For this review, take the finished solid that the model builds, in its own axes (mm). Face numbers are marked on the shaded views. Coordinates: 2 decimals unless noted, no trailing zeros. Write each loop counter-clockwise with the first axis right and the second up, starting at its lowest first coordinate (ties: lowest second). Pieces come first, ordered by that corner, then holes. Notation, with made-up numbers: (73.5, 17.25) -> (116.5, 17.25) arc R23 ccw to (116.5, 33.25) -> close; hole circle Ø4 at (32, 14.5). An arc over 180 degrees is marked (long way). Put each result on its own line as item: value. Start each with the question number.
Item 1: Consider section A-A on x = 92. Give the boundary of the cut face in (y, z) (1 decimal).
Item 2: Consider section D-D on z = 3.5. Give the boundary of the cut face in (x, y).
Item 3: To check wall thickness, follow L1, parallel to X at y = 45.5, z = -2 (3 decimals); L2, parallel to X at y = 52.5, z = -0.75; L3, parallel to Y at x = 103, z = -2.25. State the ranges of each line that lie inside material, in increasing order.
Item 4: Consider section C-C on y = 53. Give the boundary of the cut face in (x, z) (1 decimal), and give its area (3 significant figures).
Item 5: Consider section B-B on y = 42.5. Give the boundary of the cut face in (x, z) (1 decimal).
Item 6: The part is to be moulded in two halves that separate along Z. For the marked faces 1 and 2, say which applies: +Z half, -Z half, draft (parallel to the pull), parting line (faces both ways), or undercut.
Item 7: Insertion check: P1, Ø1, axis at x = 99, z = 0.5, coming from the -Y side; P2, Ø13, axis at x = 95.86, y = 45.47, coming from the -Z side; P3, Ø4, axis at y = 31, z = 2, coming from the +X side. Each pin has a flat end and moves straight along its axis. Give the tip position at first contact, or say it passes through.
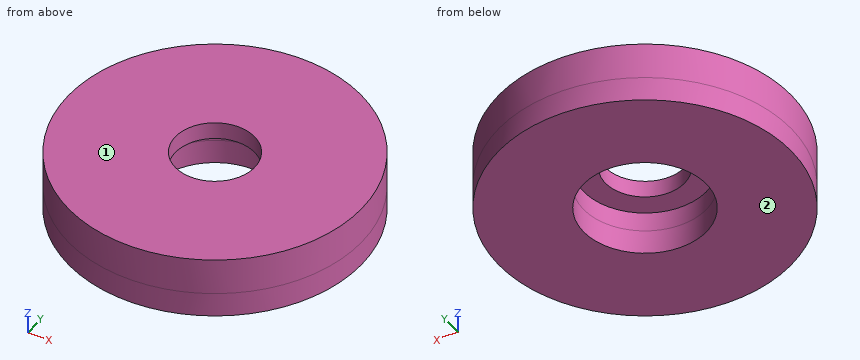
```python
from build123d import *

# Parameters (mm, degrees)
SKETCH1_R               = 19.05
SKETCH1_R_2             = 8.001
BOSS_EXTRUDE1_DEPTH     = 3.175
SKETCH2_R               = 19.05
BOSS_EXTRUDE2_DEPTH     = 4.7625
F_3_8_CLEARANCE_HOLE1_D = 10.31748
SKETCH6_R               = 8.001
CUT_EXTRUDE1_DEPTH      = 2.54


with BuildPart() as part:
    # Sketch1 → Boss-Extrude1 (new body)
    with BuildSketch(Plane.XY):
        with Locations((95.864074702, 45.465579041)):
            Circle(SKETCH1_R)
        with Locations((95.864074702, 45.465579041)):
            Circle(SKETCH1_R_2, mode=Mode.SUBTRACT)
    extrude(amount=-BOSS_EXTRUDE1_DEPTH)

    # Sketch2 → Boss-Extrude2 (add)
    with BuildSketch(Plane.XY):
        with Locations((95.864074702, 45.465579041)):
            Circle(SKETCH2_R)
    extrude(amount=BOSS_EXTRUDE2_DEPTH)

    # 3/8 Clearance Hole1 (through all)
    with Locations(Plane.XY.offset(4.7625)):
        with Locations((95.864074702, 45.465579041)):
            Hole(F_3_8_CLEARANCE_HOLE1_D / 2)

    # Sketch6 → Cut-Extrude1 (cut)
    with BuildSketch(Plane(origin=(0, 0, 0), x_dir=(-1, 0, 0), z_dir=(0, 0, -1))):
        with Locations((-95.864074702, 45.465579041)):
            Circle(SKETCH6_R)
    extrude(amount=-CUT_EXTRUDE1_DEPTH, mode=Mode.SUBTRACT)


solid = part.part
```
Return value:
1. outline: (26.8, -3.2) -> (38.5, -3.2) -> (38.5, 2.5) -> (42, 2.5) -> (42, 4.8) -> (26.8, 4.8) -> close; (48.9, 2.5) -> (52.5, 2.5) -> (52.5, -3.2) -> (64.1, -3.2) -> (64.1, 4.8) -> (48.9, 4.8) -> close
2. outline: circle Ø38.1 at (95.86, 45.47); hole circle Ø10.32 at (95.86, 45.47)
3. L1: 76.814 to 87.863, 103.865 to 114.914
3. L2: 78.16 to 92.05, 99.68 to 113.57
3. L3: 27.8 to 41.85, 49.08 to 63.13
4. outline: (78.4, -3.2) -> (93.2, -3.2) -> (93.2, 2.5) -> (98.6, 2.5) -> (98.6, -3.2) -> (113.4, -3.2) -> (113.4, 4.8) -> (78.4, 4.8) -> close
4. area: 247 mm^2
5. outline: (77, -3.2) -> (88.4, -3.2) -> (88.4, 2.5) -> (91.6, 2.5) -> (91.6, 4.8) -> (77, 4.8) -> close; (100.1, 2.5) -> (103.3, 2.5) -> (103.3, -3.2) -> (114.7, -3.2) -> (114.7, 4.8) -> (100.1, 4.8) -> close
6. face 1: +Z half
6. face 2: -Z half
7. P1: y = 26.6
7. P2: z = 2.54
7. P3: x = 110.27
